Autodesk Inventor part; units mm, degrees
ref_plane "YZ Plane" through (0, 0, 0) normal (1, 0, 0) x (0, 1, 0)
ref_plane "XZ Plane" through (0, 0, 0) normal (0, 1, 0) x (-1, 0, 0)
ref_plane "XY Plane" through (0, 0, 0) normal (0, 0, 1) x (1, 0, 0)
sketch "Sketch1" plane through (0, 0, 0) normal (0, 1, 0) x (-1, 0, 0)
  line L0 (0, 0) -> (-457.2, 0)
  line L1 (-457.2, 0) -> (-457.2, -127)
  line L2 (-457.2, -127) -> (0, -127)
  line L3 (0, -127) -> (0, 0)
  dimension "d0" = 457.2
  dimension "d1" = 127
extrude "Extrusion1" add sketch "Sketch1" along normal blind 3.175
sketch "Sketch2" plane through (0, 3.175, 0) normal (0, 1, 0) x (1, 0, 0)
  line L0 (0, 127) -> (0, 0)
  line L1 (0, 114.3) -> (25.4, 114.3)
  line L2 (25.4, 114.3) -> (25.4, 127)
  line L3 (457.2, 127) -> (0, 127)
  line L4 (63.5, 127) -> (63.5, 114.3)
  line L5 (63.5, 114.3) -> (88.9, 114.3)
  line L6 (88.9, 114.3) -> (88.9, 127)
  line L7 (127, 127) -> (127, 114.3)
  line L8 (127, 114.3) -> (152.4, 114.3)
  line L9 (152.4, 114.3) -> (152.4, 127)
  line L10 (190.5, 127) -> (190.5, 114.3)
  line L11 (190.5, 114.3) -> (215.9, 114.3)
  line L12 (215.9, 114.3) -> (215.9, 127)
  line L13 (254, 127) -> (254, 114.3)
  line L14 (254, 114.3) -> (279.4, 114.3)
  line L15 (279.4, 114.3) -> (279.4, 127)
  line L16 (317.5, 127) -> (317.5, 114.3)
  line L17 (317.5, 114.3) -> (342.9, 114.3)
  line L18 (342.9, 114.3) -> (342.9, 127)
  line L19 (381, 127) -> (381, 114.3)
  line L20 (381, 114.3) -> (406.4, 114.3)
  line L21 (406.4, 114.3) -> (406.4, 127)
  line L22 (444.5, 127) -> (444.5, 114.3)
  line L23 (444.5, 114.3) -> (457.2, 114.3)
  line L24 (457.2, 0) -> (457.2, 127)
  line L25 (0, 114.3) -> (0, 127)
  line L26 (63.5, 127) -> (88.9, 127)
  line L27 (127, 127) -> (152.4, 127)
  line L28 (190.5, 127) -> (215.9, 127)
  line L29 (254, 127) -> (279.4, 127)
  line L30 (317.5, 127) -> (342.9, 127)
  line L31 (381, 127) -> (406.4, 127)
  line L32 (444.5, 127) -> (457.2, 127)
  line L33 (0, 127) -> (25.4, 127)
  point P0 (457.2, 114.3)
  point P1 (25.4, 127)
  dimension "d4" = 25.4
  dimension "d6" = 12.7
  dimension "d7" = 12.7
  dimension "d8" = 12.7
  dimension "d9" = 25.4
  dimension "d10" = 38.1
  dimension "d11" = 25.4
  dimension "d12" = 38.1
  dimension "d13" = 25.4
  dimension "d14" = 38.1
  dimension "d15" = 25.4
  dimension "d16" = 38.1
  dimension "d17" = 25.4
  dimension "d18" = 38.1
  dimension "d19" = 25.4
  dimension "d20" = 38.1
  dimension "d21" = 12.7
  dimension "d22" = 0
  dimension "d42" = 12.7
extrude "Extrusion2" cut sketch "Sketch2" against normal through all
sketch "Sketch3" plane through (0, 3.175, 0) normal (0, 1, 0) x (1, 0, 0)
  line L0 (0, 0) -> (457.2, 0)
  line L1 (0, 0) -> (25.4, 0)
  line L2 (25.4, 0) -> (25.4, 12.7)
  line L3 (25.4, 12.7) -> (0, 12.7)
  line L4 (0, 12.7) -> (0, 0)
  line L5 (63.5, 0) -> (88.9, 0)
  line L6 (88.9, 0) -> (88.9, 12.7)
  line L7 (88.9, 12.7) -> (63.5, 12.7)
  line L8 (63.5, 12.7) -> (63.5, 0)
  line L9 (127, 0) -> (152.4, 0)
  line L10 (152.4, 0) -> (152.4, 12.7)
  line L11 (152.4, 12.7) -> (127, 12.7)
  line L12 (127, 12.7) -> (127, 0)
  line L13 (190.5, 0) -> (215.9, 0)
  line L14 (215.9, 0) -> (215.9, 12.7)
  line L15 (215.9, 12.7) -> (190.5, 12.7)
  line L16 (190.5, 12.7) -> (190.5, 0)
  line L17 (254, 0) -> (279.4, 0)
  line L18 (279.4, 0) -> (279.4, 12.7)
  line L19 (279.4, 12.7) -> (254, 12.7)
  line L20 (254, 12.7) -> (254, 0)
  line L21 (317.5, 0) -> (342.9, 0)
  line L22 (342.9, 0) -> (342.9, 12.7)
  line L23 (342.9, 12.7) -> (317.5, 12.7)
  line L24 (317.5, 12.7) -> (317.5, 0)
  line L25 (381, 0) -> (406.4, 0)
  line L26 (406.4, 0) -> (406.4, 12.7)
  line L27 (406.4, 12.7) -> (381, 12.7)
  line L28 (381, 12.7) -> (381, 0)
  line L29 (457.2, 0) -> (457.2, 114.3)
  line L30 (457.2, 0) -> (444.5, 0)
  line L31 (444.5, 0) -> (444.5, 12.7)
  line L32 (444.5, 12.7) -> (457.2, 12.7)
  line L33 (457.2, 12.7) -> (457.2, 0)
  dimension "d25" = 25.4
  dimension "d26" = 12.7
  dimension "d27" = 25.4
  dimension "d28" = 38.1
  dimension "d29" = 25.4
  dimension "d30" = 25.4
  dimension "d31" = 25.4
  dimension "d32" = 25.4
  dimension "d33" = 25.4
  dimension "d34" = 12.7
  dimension "d35" = 38.1
  dimension "d36" = 38.1
  dimension "d37" = 38.1
  dimension "d38" = 38.1
  dimension "d39" = 38.1
extrude "Extrusion3" cut sketch "Sketch3" against normal through all
properties part number "BridgeRoof"
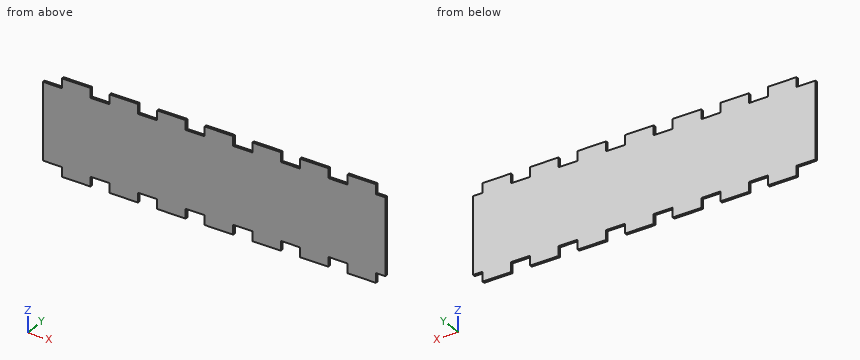
Source: CAD feature listing. Evaluate the final solid. Frame: model axes, mm. Round coordinates to 2 decimals unless told otherwise and drop trailing zeros. Write each loop counter-clockwise with the first axis right and the second up, starting at its lowest first coordinate (ties: lowest second). Pieces come first, ordered by that corner, then holes. Notation, with made-up numbers: (-7.5, -17.75) - (13.5, -17.75) arc R21 cw to (13.5, -10.75) - close; hole circle Ø3 at (85.5, 80). An arc over 180 degrees is marked (long way). Use CSV: the item, a comma, the result in double quotes. Start each with the question number.
(1) First-contact query: pin 1 Ø1 at (x, y) = (268, 2.5) entering from +Z; pin 2 Ø1.6 at (y, z) = (1, -119.5) entering from -X; pin 3 Ø1 at (x, y) = (447.5, 2) entering from -Z. Flat tips, straight axial feed; report the tip coordinate or a pass-through.
(2) Material intervals for probe 1 along Z at (x, y) = (128.5, 2.2), sorted ascending. Write a range as [from, to].
(3) Cut plane A-A, the plane x = 208. Return loops of the section in (y, z) (3 decimals).
Geometry says:
1,pin 1,"z = -12.7"
1,pin 2,"x = 25.4"
1,pin 3,"z = -114.3"
2,probe 1,"[-114.3, -12.7]"
3,outline,"(0, -114.3) - (3.175, -114.3) - (3.175, -12.7) - (0, -12.7) - close"
